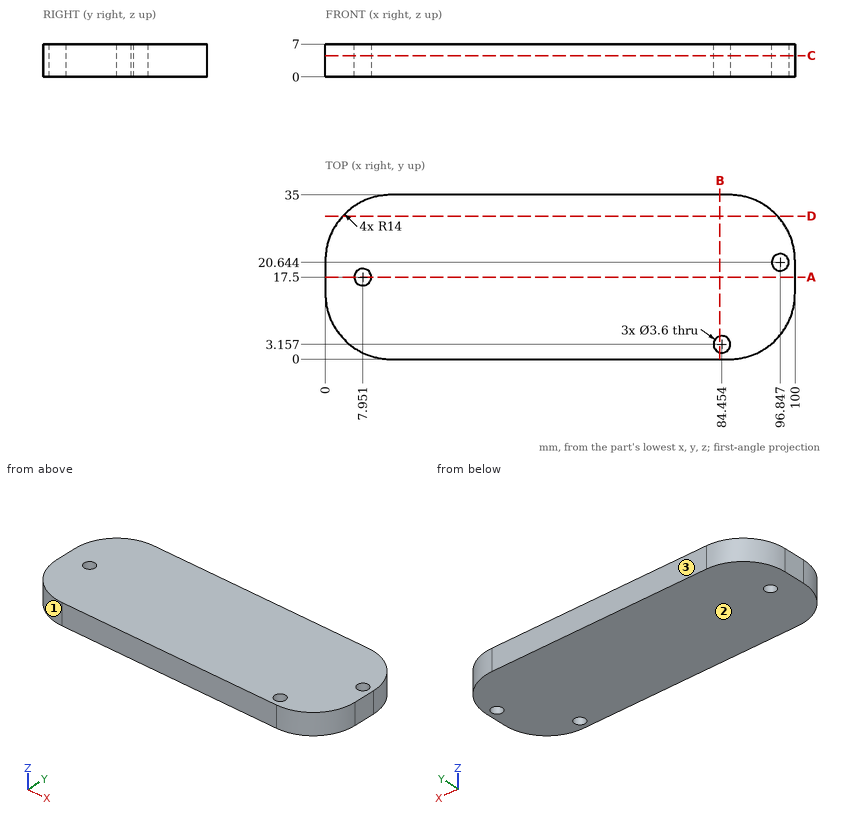
Here's the drawing with two shaded views (mm, measured from the low corner). I have some questions. Coordinates: 2 decimals unless noted, no trailing zeros. Order: outer loops, then holes, each group sorted by start corner. A loop starts at its lowest first (then second) coordinate and runs counter-clockwise, first axis right, second up.
Q1. Suppose I cut it at B-B on x = 84. Please give me the cut outline in (y, z) (1 decimal), and give its area (3 significant figures).
Q2. Will these pins go through, and if not, where does the flat tip stop? pin 1 (1 mm diameter, centred on y = 6, z = 4.5, fed in from +X); pin 2 (4 mm diameter, centred on y = 27, z = 5.5, fed in from -X).
Q3. Please list where these lines run through material, in increasing order: L1, parallel to X at y = 20.5, z = 5; L2, parallel to Y at x = 96, z = 4.75 (1 decimal); L3, parallel to X at y = 16, z = 1.75 (1 decimal).
Q4. Suppose I cut it at D-D on y = 30.5. Please give me the cut outline in (x, z).
Q5. Suppose I cut it at C-C on z = 4.5. Please give me the cut outline in (x, y), and give its area (3 significant figures).
Q6. Suppose I cut it at A-A on y = 17.5. Please give me the cut outline in (x, z).
Q7. Thinking about a two-plate mould opening in Y: for the marked faces 1, 2 and 3, which applies, released by +Y, released by -Y, zero draft, split by the parting line, or undercut?
Answer:
1. outline: (0, 0) - (1.4, 0) - (1.4, 7) - (0, 7) - close; (4.9, 0) - (35, 0) - (35, 7) - (4.9, 7) - close
1. area: 221 mm2
2. pin 1: stops at x = 97.82
2. pin 2: stops at x = 0.58
3. L1: x = 0 to 95.05, 98.64 to 100
3. L2: y = 4.2 to 19.1, 22.2 to 30.8
3. L3: x = 0 to 7, 8.9 to 100
4. outline: (3.72, 0) - (96.28, 0) - (96.28, 7) - (3.72, 7) - close
5. outline: (0, 14) arc R14 ccw to (14, 0) - (86, 0) arc R14 ccw to (100, 14) - (100, 21) arc R14 ccw to (86, 35) - (14, 35) arc R14 ccw to (0, 21) - close; hole circle Ø3.6 at (7.95, 17.5); hole circle Ø3.6 at (84.45, 3.16); hole circle Ø3.6 at (96.85, 20.64)
5. area: 3,300 mm2
6. outline: (0, 0) - (6.15, 0) - (6.15, 7) - (0, 7) - close; (9.75, 0) - (100, 0) - (100, 7) - (9.75, 7) - close
7. face 1: released by -Y
7. face 2: zero draft
7. face 3: released by +Y
